Build history of the part. All positions in model axes, mm. Face numbers are marked on the shaded views. A direction names the side the tool comes from. Give positions to 0.01 mm unless a question says otherwise; leave off trailing zeros. Write each loop counter-clockwise with the first axis right and the second up, starting at its lowest first coordinate (ties: lowest second). Pieces come first, ordered by that corner, then holes. Notation, with made-up numbers: M 81,36 L 102,36 A24 cw 102,58 Z; hole C 50,82.5 d1. An arc over 180 degrees is marked long. Return JSON: item names as keys, results as strings. Group by question number.
Q1. Flat gauge pins, fed straight in: pin 1 Ø3 at (x, z) = (-9, -9.5) entering from -Y; pin 2 Ø3 at (y, z) = (8, 11) entering from +X; pin 3 Ø2 at (x, y) = (18, 4.5) entering from +Z; pin 4 Ø3 at (x, z) = (16.5, 19) entering from +Y. Where does each tip first touch, or does it go through?
Q2. Pull direction Y, two halves, no side cores. Call the marked faces 4, 5 and 6: +Y half, -Y half, draft (parallel to the pull), parting line (faces both ways), or undercut.
Q3. Band-saw the part on B-B, the plane y = -4.75. Give the cut face in (x, z).
Q4. Tool access for the marked faces 1, 2 and 3: list every direction of +Z, -Z, +X, -X, +Y, -Y with a clear straight run to the whole face (end or side of a thin tool).
Q5. Band-saw the part on A-A, the plane y = 13.75. Give the cut face in (x, z).
Q6. Wall check: probe 1 along X at (y, z) = (19.9, 0); probe 2 along Y at (x, z) = (-1.5, 16); probe 3 along Y at (x, z) = (-1.5, 1.5). Give the ranges that are in metal, low to high.
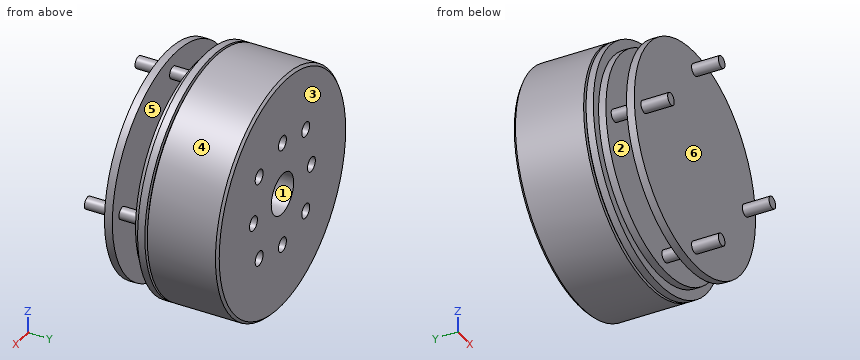
from build123d import *

# Parameters (mm, degrees)
SKETCH_2_R          = 1.5
CUT_EXTRUDE_1_DEPTH = 3
SKETCH_3_R          = 4.25
CUT_EXTRUDE_2_DEPTH = 18
SKETCH_6_R          = 1.25
EXTRUDE_1_DEPTH     = 4.5
SKETCH_7_R          = 23
EXTRUDE_2_DEPTH     = 1.6
SKETCH_10_R         = 1.25
EXTRUDE_3_DEPTH     = 5.5


with BuildPart() as part:
    # 草图1 → 旋转1 (revolve)
    with BuildSketch(Plane.XY, mode=Mode.PRIVATE) as revolve_1_sk:
        Polygon((24, 22.1), (0, 22.1), (0, 4.545296676), (0, 3.1), (8.3, 3.1), (8.3, 4.1), (22.5, 4.1), (22.5, 5.6), (24.5, 5.6), (24.5, 7.1), (23.5, 7.1), (23.5, 7.6), (24.5, 7.6), (24.5, 21.6), align=None)
    revolve(revolve_1_sk.sketch.rotate(Axis((0, 4.545296676, 0), (0, 1, 0)), 90), axis=Axis((0, 4.545296676, 0), (0, 1, 0)))

    # 草图2 → 切除-拉伸1 (cut)
    with BuildSketch(Plane(origin=(0, 22.1, 0), x_dir=(1, 0, 0), z_dir=(0, 1, 0))):
        with Locations(Location((0, 11, 0), (0, 0, 270))):
            Circle(SKETCH_2_R)
        with Locations(Location((11, 0, 0), (0, 0, 270))):
            Circle(SKETCH_2_R)
        with Locations(Location((0, -11, 0), (0, 0, 270))):
            Circle(SKETCH_2_R)
        with Locations(Location((-11, 0, 0), (0, 0, 270))):
            Circle(SKETCH_2_R)
        with Locations(Location((8.838834765, 8.838834765, 0), (0, 0, 270))):
            Circle(SKETCH_2_R)
        with Locations(Location((8.838834765, -8.838834765, 0), (0, 0, 270))):
            Circle(SKETCH_2_R)
        with Locations(Location((-8.838834765, -8.838834765, 0), (0, 0, 270))):
            Circle(SKETCH_2_R)
        with Locations(Location((-8.838834765, 8.838834765, 0), (0, 0, 270))):
            Circle(SKETCH_2_R)
    extrude(amount=-CUT_EXTRUDE_1_DEPTH, mode=Mode.SUBTRACT)

    # 草图3 → 切除-拉伸2 (cut)
    with BuildSketch(Plane(origin=(0, 22.1, 0), x_dir=(1, 0, 0), z_dir=(0, 1, 0))):
        with Locations(Location((0, 0, 0), (0, 0, 270))):
            Circle(SKETCH_3_R)
    extrude(amount=-CUT_EXTRUDE_2_DEPTH, mode=Mode.SUBTRACT)

    # 草图6 → 凸台-拉伸1 (add)
    with BuildSketch(Plane.XZ.offset(-4.1)):
        with Locations(Location((0, 19.25, 0), (0, 0, 270))):
            Circle(SKETCH_6_R)
        with Locations(Location((19.25, 0, 0), (0, 0, 270))):
            Circle(SKETCH_6_R)
        with Locations(Location((0, -19.25, 0), (0, 0, 270))):
            Circle(SKETCH_6_R)
        with Locations(Location((-19.25, 0, 0), (0, 0, 270))):
            Circle(SKETCH_6_R)
    extrude(amount=EXTRUDE_1_DEPTH)

    # 草图7 → 凸台-拉伸2 (add)
    with BuildSketch(Plane.XZ.offset(0.4)):
        with Locations(Location((0, 0, 0), (0, 0, 270))):
            Circle(SKETCH_7_R)
    extrude(amount=EXTRUDE_2_DEPTH)

    # 草图10 → 凸台-拉伸3 (add)
    with BuildSketch(Plane.XZ.offset(2)):
        with Locations(Location((0, 19.25, 0), (0, 0, 270))):
            Circle(SKETCH_10_R)
        with Locations(Location((19.25, 0, 0), (0, 0, 270))):
            Circle(SKETCH_10_R)
        with Locations(Location((0, -19.25, 0), (0, 0, 270))):
            Circle(SKETCH_10_R)
        with Locations(Location((-19.25, 0, 0), (0, 0, 270))):
            Circle(SKETCH_10_R)
    extrude(amount=EXTRUDE_3_DEPTH)


solid = part.part
From the geometry:
{
 "1": {"pin 1": "stops at y = -2", "pin 2": "stops at x = 22.58", "pin 3": "stops at z = 14.74", "pin 4": "stops at y = 22.1"},
 "2": {"face 4": "draft", "face 5": "undercut", "face 6": "-Y half"},
 "3": {"outline": "C -19.25,0 d2.5; C 0,-19.25 d2.5; C 0,19.25 d2.5; C 19.25,0 d2.5"},
 "4": {"face 1": "+Y", "face 2": "none", "face 3": "+Z, -Z, +X, -X, +Y"},
 "5": {"outline": "C 0,0 d49; hole C 0,0 d8.5"},
 "6": {"probe 1": "x = -24.5 to -12.5, -9.5 to -4.25, 4.25 to 9.5, 12.5 to 24.5", "probe 2": "y = -2 to -0.4, 4.1 to 22.1", "probe 3": "y = -2 to -0.4, 3.1 to 4.1"}
}
